Check sheet for the modelled part. Datum: model origin and axes. Units: mm. Give positions to 0.01 mm unless a question says otherwise; leave off trailing zeros. Order: outer loops, then holes, each group sorted by start corner. A loop starts at its lowest first (then second) coordinate and runs counter-clockwise, first axis right, second up. Notation, with made-up numbers: (85.5, 47) -> (144.5, 47) arc R24 ccw to (144.5, 77) -> close; hole circle Ø2 at (78.25, 41). An arc over 180 degrees is marked (long way). One line per question, with ' | ' between items.
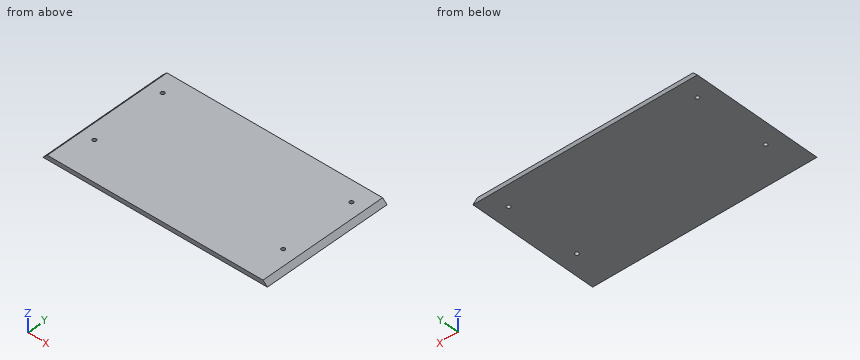
Autodesk Inventor part; units mm, degrees
ref_plane "YZ Plane" through (0, 0, 0) normal (1, 0, 0) x (0, 1, 0)
ref_plane "XZ Plane" through (0, 0, 0) normal (0, 1, 0) x (-1, 0, 0)
ref_plane "XY Plane" through (0, 0, 0) normal (0, 0, 1) x (1, 0, 0)
sketch "Sketch1" plane through (0, 0, 0) normal (0, 0, 1) x (1, 0, 0)
  line L0 (0, 0) -> (208, 0)
  line L1 (208, 0) -> (208, -121)
  line L2 (208, -121) -> (0, -121)
  line L3 (0, -121) -> (0, 0)
  dimension "d0" = 208
  dimension "d1" = 121
extrude "Extrusion1" add sketch "Sketch1" along normal blind 4
sketch "Sketch2" plane through (0, 0, 0) normal (0, 0, -1) x (-1, 0, 0)
  line L0 (0, -121) -> (-208, -121)
  line L1 (0, -121) -> (-16.5, -121)
  line L2 (-16.5, -121) -> (-16.5, -87)
  line L3 (-16.5, -87) -> (0, -87)
  line L4 (0, -87) -> (0, -121)
  point P0 (0, 0)
  dimension "d4" = 16.5
  dimension "d5" = 34
hole "Hole1" at (16.5, -87, 0) direction (0, 0, 1) diameter 3.5 depth 8.8
ref_plane "Work Plane1" through (104, -121, 0) normal (-1, 0, 0) x (0, 0, 1)
ref_plane "Work Plane2" through (0, -60.5, 0) normal (0, 1, 0) x (1, 0, 0)
sketch "Sketch3" plane through (0, 0, 4) normal (0, 0, 1) x (1, 0, 0)
  line L0 (208, 0) -> (0, 0)
  line L1 (0, 0) -> (16.5, 0)
  line L2 (16.5, 0) -> (16.5, -18)
  line L3 (16.5, -18) -> (0, -18)
  line L4 (0, -18) -> (0, 0)
  dimension "d13" = 16.5
  dimension "d14" = 18
hole "Hole2" at (16.5, -18, 4) direction (0, 0, -1) diameter 3.5 depth 8.8
mirror "Mirror1" about plane through (104, -121, 0) normal (-1, 0, 0) of "Hole2", "Hole1"
chamfer "Chamfer1" distance 4 angle 45 2 edges at (0, -60.5, 4) (208, -60.5, 4)
properties part number "wall-front"
Q1. Section check A-A (z = 2.45). Enter the section's corners in (x, y).
Result sheet:
outline: (2.45, -121) -> (205.55, -121) -> (205.55, 0) -> (2.45, 0) -> close; hole circle Ø3.5 at (16.5, -87); hole circle Ø3.5 at (16.5, -18); hole circle Ø3.5 at (191.5, -87); hole circle Ø3.5 at (191.5, -18)
Q2. Thickness scan on line 1 (Y direction, x = 16.5, z = 0.95); line 2 (X direction, y = -18, z = 1.65); line 3 (X direction, y = -18, z = 1.7). Record the ranges inside material, lowest first.
Result sheet:
line 1: y = -121 to -88.75, -85.25 to -19.75, -16.25 to 0 | line 2: x = 1.65 to 14.75, 18.25 to 189.75, 193.25 to 206.35 | line 3: x = 1.7 to 14.75, 18.25 to 189.75, 193.25 to 206.3
Q3. Depth check by flat-ended pin: pin 1 Ø2 at (x, y) = (16.5, -18) entering from +Z; pin 2 Ø2 at (y, z) = (-99, 3.5) entering from +X; pin 3 Ø1.5 at (y, z) = (-52.5, 2) entering from -X. Enter the tip coordinate at first touch or a pass-through.
Result sheet:
pin 1: passes through | pin 2: stops at x = 205.5 | pin 3: stops at x = 1.25
